For this review, use the dimensioned drawing (mm, ordinates from the lowest corner) and the shaded views. A direction names the side the tool comes from. Coordinates: 2 decimals unless noted, no trailing zeros. Write each loop counter-clockwise with the first axis right and the second up, starting at its lowest first coordinate (ties: lowest second). Pieces come first, ordered by that corner, then holes. Notation, with made-up numbers: (-21, -14.75) - (3, -14.75) arc R24 ccw to (3, 4.25) - close; hole circle Ø9 at (61, -38). An arc over 180 degrees is marked (long way). Answer as a JSON object with one key per item and string values.
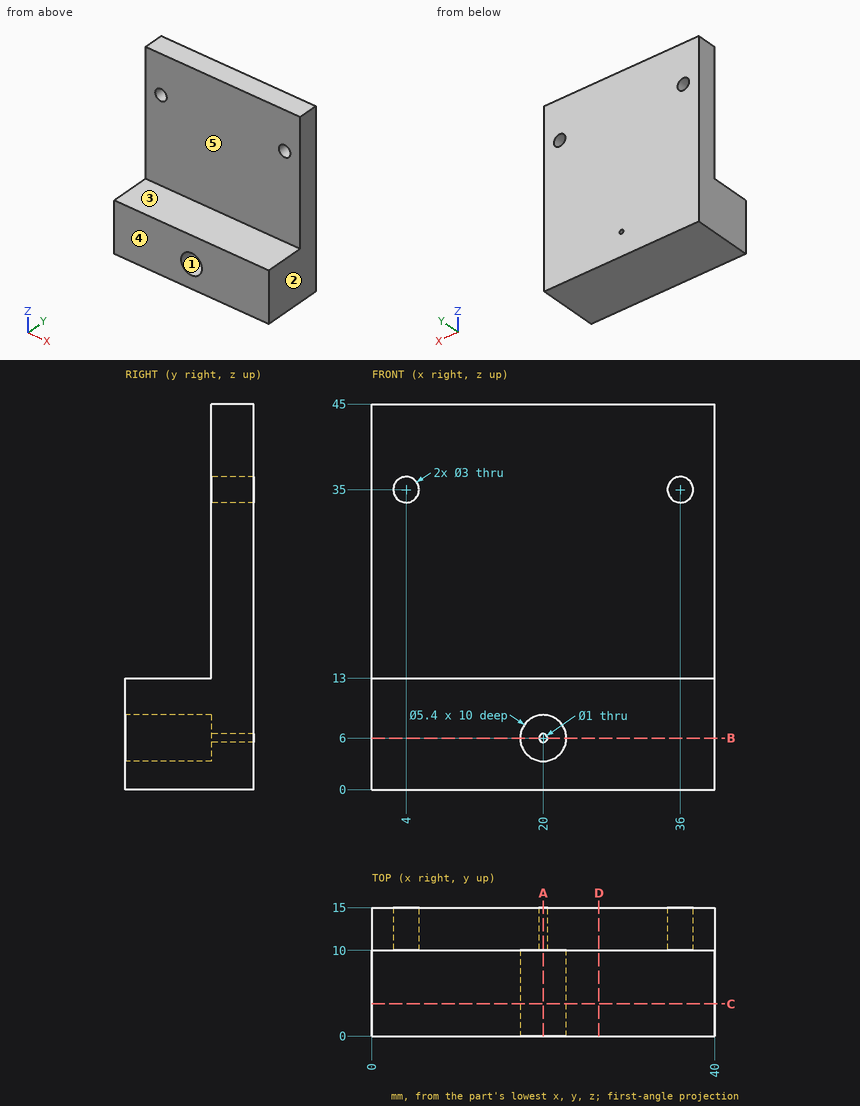
(1) Take a section at D-D, the plane x = 26.5. Write out the cut boundary in (y, z), and give its area (3 significant figures).
Solved:
{"outline": "(0, 0) - (15, 0) - (15, 45) - (10, 45) - (10, 13) - (0, 13) - close", "area": "355 mm^2"}
(2) For pin 1 (5 mm diameter, centred on x = 36, z = 35, fed in from -Y); pin 2 (8 mm diameter, centred on x = 19.5, y = 5.5, fed in from +Z), all flat-tipped, find the tip position at first contact; note any pin that passes through.
Solved:
{"pin 1": "stops at y = 10", "pin 2": "stops at z = 13"}
(3) The part is to be moulded in two halves that separate along Z. For the marked faces 1, 2 and 3, say which applies: pulls with the +Z half, pulls with the -Z half, needs draft (parallel to the pull), parting line crosses it, or undercut.
Solved:
{"face 1": "undercut", "face 2": "needs draft", "face 3": "pulls with the +Z half"}
(4) To check wall thickness, follow line 1 (Z direction, x = 20, y = 2.5); line 2 (Z direction, x = 36, y = 11.55); line 3 (Y direction, x = 23.5, z = 20.5). State the ranges of each line that lie inside material, in increasing order. Write a range as from..to.
Solved:
{"line 1": "z = 0..3.3, 8.7..13", "line 2": "z = 0..33.5, 36.5..45", "line 3": "y = 10..15"}
(5) Take a section at B-B, the plane z = 6. Write out the cut boundary in (x, y).
Solved:
{"outline": "(0, 0) - (17.3, 0) - (17.3, 10) - (19.5, 10) - (19.5, 15) - (0, 15) - close; (20.5, 10) - (22.7, 10) - (22.7, 0) - (40, 0) - (40, 15) - (20.5, 15) - close"}
(6) Tool access review of the marked faces 4 and 5: name each direction out of +Z, -Z, +X, -X, +Y, -Y from which nothing blocks a thin tool from reaching the whole face with its end or side.
Solved:
{"face 4": "+Z, -Z, +X, -X, -Y", "face 5": "+Z, +X, -X, -Y"}
(7) Take a section at A-A, the plane x = 20. Write out the cut boundary in (y, z), and give its area (3 significant figures).
Solved:
{"outline": "(0, 0) - (15, 0) - (15, 5.5) - (10, 5.5) - (10, 3.3) - (0, 3.3) - close; (0, 8.7) - (10, 8.7) - (10, 6.5) - (15, 6.5) - (15, 45) - (10, 45) - (10, 13) - (0, 13) - close", "area": "296 mm^2"}
(8) Take a section at C-C, the plane y = 3.75. Write out the cut boundary in (x, z).
Solved:
{"outline": "(0, 0) - (40, 0) - (40, 13) - (0, 13) - close; hole circle Ø5.4 at (20, 6)"}
